Can you work these out from the model? Positions are in its coordinate system, mm. Face numbers are marked on the shaded views. A direction names the side the tool comes from. Coordinates: 2 decimals unless noted, no trailing zeros. Order: outer loops, then holes, each group sorted by start corner. A loop starts at its lowest first (then second) coordinate and runs counter-clockwise, first axis right, second up. Notation, with made-up numbers: (23.5, 1.5) -> (34.5, 1.5) arc R25 ccw to (34.5, 33.5) -> close; hole circle Ø6 at (23.25, -19.5). An arc over 180 degrees is marked (long way). Write item = value, one per line.
```python
from build123d import *

# Parameters (mm, degrees)
F1_DEPTH = 50.8
F3_DEPTH = 28.575003
F4_W     = 101.6
F4_H     = 58.923625
F4_R     = 12.7
F5_DEPTH = 25.4


with BuildPart() as f1:
    # F0 (on Front) → F1 (new body, symmetric)
    with BuildSketch(Plane.XZ):
        Polygon((17.145002, -15.174311), (17.145002, 43.749314), (-17.145002, 43.749314), (-17.145002, -15.174311), (-71.733102, -15.174311), (-71.733102, -43.749314), (-17.145002, -43.749314), (17.145002, -43.749314), align=None)
    extrude(amount=F1_DEPTH, both=True)

    # F2 (on face) → F3 (cut, through all)
    with BuildSketch(Plane.XY.offset(-15.174311)):
        with BuildLine():
            ThreePointArc((-37.474338, -8.679342), (-46.153679, 0), (-37.474338, 8.679342))
            Line((-37.474338, 8.679342), (-71.733102, 8.679342))
            Line((-71.733102, 8.679342), (-71.733102, -8.679342))
            Line((-71.733102, -8.679342), (-37.474338, -8.679342))
        make_face()
        with BuildLine():
            ThreePointArc((-37.474338, -8.679342), (-31.337117, -6.137221), (-28.794996, 0))
            ThreePointArc((-28.794996, 0), (-31.337117, 6.137221), (-37.474338, 8.679342))
            ThreePointArc((-37.474338, 8.679342), (-46.153679, 0), (-37.474338, -8.679342))
        make_face()
    extrude(amount=-F3_DEPTH, mode=Mode.SUBTRACT)

    # F4 (on face) → F5 (join)
    with BuildSketch(Plane(origin=(-17.145002, 0, 0), x_dir=(0, -1, 0), z_dir=(-1, 0, 0))):
        with Locations((0, 14.287501)):
            Rectangle(F4_W, F4_H)
        with Locations((0, 17.426297)):
            Circle(F4_R, mode=Mode.SUBTRACT)
    extrude(amount=F5_DEPTH)


solid = f1.part
```
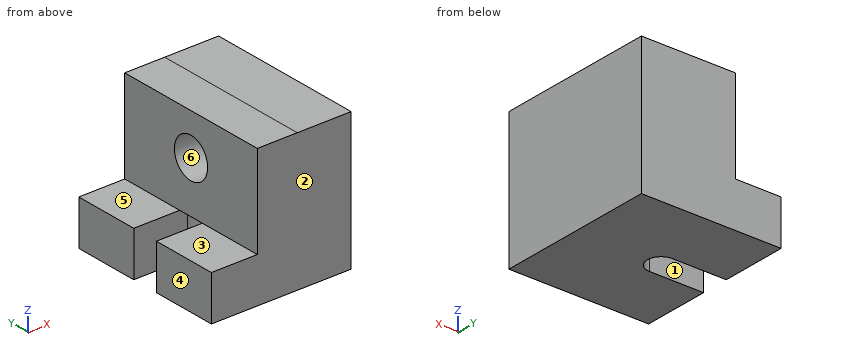
Item 1: If I drill on probe 1 along Z at (x, y) = (-24, 0); probe 2 along Z at (x, y) = (-34.25, 0); probe 3 along Z at (x, y) = (-65, 29), over which ranges is the centre line in solid material (lowest first)?
A:
probe_1 = -43.75 to 4.73, 30.13 to 43.75
probe_2 = -15.17 to 4.73, 30.13 to 43.75
probe_3 = -43.75 to -15.17
Item 2: If we mould it in two halves opening along Y, with no side actions, what happens to the marked faces 1, 2 and 3? For each: pulls with the +Y half, pulls with the -Y half, needs draft (parallel to the pull), parting line crosses it, or undercut.
A:
face_1 = undercut
face_2 = pulls with the -Y half
face_3 = needs draft
Item 3: I'm going to push flat-ended pins straight in: P1, Ø9, axis at x = -58.5, y = -28.5, coming from the +Z side; P2, Ø23, axis at y = 0, z = 17.43, coming from the -X side (3 decimals); P3, Ø8, axis at y = -1.5, z = 3, coming from the -X side (3 decimals). Where does each tip first touch, or does it pass through?
A:
P1 = -15.17
P2 = -17.145
P3 = -42.545
Item 4: For the marked faces 4, 5 and 6, which set-ups out of +Z, -Z, +X, -X, +Y, -Y let a thin tool reach every point of the face, with its end or its side?
A:
face_4 = +Z, -Z, -X, +Y, -Y
face_5 = +Z, -X, +Y, -Y
face_6 = -X
Item 5: I want a section at C-C, the plane y = -5. Please give me the cut outline in (x, z) (3 decimals).
A:
outline = (-42.545, -15.174) -> (-30.38, -15.174) -> (-30.38, -43.749) -> (17.145, -43.749) -> (17.145, 43.749) -> (-42.545, 43.749) -> (-42.545, 29.101) -> (-17.145, 29.101) -> (-17.145, 5.752) -> (-42.545, 5.752) -> close
Item 6: I want a section at A-A, the plane x = -56.5. Please give me the cut outline in (y, z), plus the area to 3 significant figures.
A:
outline = (-50.8, -43.75) -> (-8.68, -43.75) -> (-8.68, -15.17) -> (-50.8, -15.17) -> close; (8.68, -43.75) -> (50.8, -43.75) -> (50.8, -15.17) -> (8.68, -15.17) -> close
area = 2,410 mm2
Item 7: I want a section at B-B, the plane z = -26. Please give me the cut outline in (x, y) (3 decimals).
A:
outline = (-71.733, -50.8) -> (17.145, -50.8) -> (17.145, 50.8) -> (-71.733, 50.8) -> (-71.733, 8.679) -> (-37.474, 8.679) arc R8.679 cw to (-28.795, 0) arc R8.679 cw to (-37.474, -8.679) -> (-71.733, -8.679) -> close
Item 8: I want a section at D-D, the plane z = 3. Please give me the cut outline in (x, y) (3 decimals).
A:
outline = (-42.545, -50.8) -> (17.145, -50.8) -> (17.145, 50.8) -> (-42.545, 50.8) -> close
